Could you check a few things on this model? Use its own coordinates, in mm. Round coordinates to 2 decimals unless told otherwise and drop trailing zeros.
from build123d import *

# Parameters (mm, degrees)
F1_DEPTH = 4


# Not quite as in the source:
# - ends of sketch curves that miss each other by under 0.0002 mm in the source are joined


with BuildPart() as f1:
    # F0 (on Top) → F1 (new body)
    with BuildSketch(Plane.XY):
        with BuildLine():
            add(Edge.make_bspline(
                [(-23.29275, 188.71263), (-40.744167, 195.27633), (-59.410257, 198.41332), (-78.043821, 198.249744)],
                knots=[0, 0, 0, 0, 1, 1, 1, 1], degree=3))
            add(Edge.make_bspline(
                [(-78.043821, 198.249744), (-119.036105, 197.889891), (-160.001254, 181.57068), (-187.364696, 150.031637)],
                knots=[0, 0, 0, 0, 1, 1, 1, 1], degree=3))
            add(Edge.make_bspline(
                [(-187.364696, 150.031637), (-187.364865, 150.031442), (-187.364978, 150.031355), (-187.365261, 150.031072)],
                knots=[0, 0, 0, 0, 1, 1, 1, 1], degree=3))
            add(Edge.make_bspline(
                [(-187.365261, 150.031072), (-223.157197, 108.912672), (-239.83493, 53.349791), (-240.796196, -0.140351)],
                knots=[0, 0, 0, 0, 1, 1, 1, 1], degree=3))
            add(Edge.make_bspline(
                [(-240.796196, -0.140351), (-240.797267, -0.200062), (-240.797267, -0.259787), (-240.796196, -0.319498)],
                knots=[0, 0, 0, 0, 1, 1, 1, 1], degree=3))
            add(Edge.make_bspline(
                [(-240.796196, -0.319498), (-239.840937, -53.821863), (-222.970632, -108.900151), (-187.197127, -149.997041)],
                knots=[0, 0, 0, 0, 1, 1, 1, 1], degree=3))
            add(Edge.make_bspline(
                [(-187.197127, -149.997041), (-147.436926, -195.824596), (-79.112374, -209.648856), (-23.30153, -188.74031)],
                knots=[0, 0, 0, 0, 1, 1, 1, 1], degree=3))
            Line((-23.30153, -188.74031), (-23.130102, -188.679124))
            add(Edge.make_bspline(
                [(-23.130102, -188.679124), (1.059853, -180.570344), (21.278733, -165.037933), (38.938938, -147.973536)],
                knots=[0, 0, 0, 0, 1, 1, 1, 1], degree=3))
            add(Edge.make_bspline(
                [(38.938938, -147.973536), (52.026993, -136.892306), (62.204773, -123.641634), (75.896277, -117.517243)],
                knots=[0, 0, 0, 0, 1, 1, 1, 1], degree=3))
            add(Edge.make_bspline(
                [(75.896277, -117.517243), (83.85737, -115.06047), (91.397501, -116.61066), (99.542858, -119.902331)],
                knots=[0, 0, 0, 0, 1, 1, 1, 1], degree=3))
            add(Edge.make_bspline(
                [(99.542858, -119.902331), (107.756908, -123.2218), (116.195437, -128.328386), (125.148457, -131.870331)],
                knots=[0, 0, 0, 0, 1, 1, 1, 1], degree=3))
            add(Edge.make_bspline(
                [(125.148457, -131.870331), (132.727224, -134.996817), (140.627979, -137.381228), (148.394876, -139.826571)],
                knots=[0, 0, 0, 0, 1, 1, 1, 1], degree=3))
            add(Edge.make_bspline(
                [(148.394876, -139.826571), (148.394876, -139.826853), (148.397698, -139.826853), (148.397698, -139.826571)],
                knots=[0, 0, 0, 0, 1, 1, 1, 1], degree=3))
            add(Edge.make_bspline(
                [(148.397698, -139.826571), (148.40052, -139.826571), (148.401649, -139.829393), (148.403907, -139.829393)],
                knots=[0, 0, 0, 0, 1, 1, 1, 1], degree=3))
            add(Edge.make_bspline(
                [(148.403907, -139.829393), (172.528911, -147.473466), (202.043599, -149.701441), (222.443157, -131.039695)],
                knots=[0, 0, 0, 0, 1, 1, 1, 1], degree=3))
            Line((222.443157, -131.039695), (222.513713, -130.980174))
            add(Edge.make_bspline(
                [(222.513713, -130.980174), (229.464818, -125.631639), (234.197007, -117.510187), (235.635381, -108.839502)],
                knots=[0, 0, 0, 0, 1, 1, 1, 1], degree=3))
            add(Edge.make_bspline(
                [(235.635381, -108.839502), (237.078806, -100.138393), (234.900785, -90.513402), (227.492818, -83.846297)],
                knots=[0, 0, 0, 0, 1, 1, 1, 1], degree=3))
            add(Edge.make_bspline(
                [(227.492818, -83.846297), (227.400465, -83.76321), (227.305045, -83.683596), (227.206758, -83.607622)],
                knots=[0, 0, 0, 0, 1, 1, 1, 1], degree=3))
            add(Edge.make_bspline(
                [(227.206758, -83.607622), (220.687876, -78.567613), (213.176701, -75.418408), (207.090691, -71.705791)],
                knots=[0, 0, 0, 0, 1, 1, 1, 1], degree=3))
            add(Edge.make_bspline(
                [(207.090691, -71.705791), (201.005472, -67.993635), (196.586267, -64.15215), (194.627165, -57.863121)],
                knots=[0, 0, 0, 0, 1, 1, 1, 1], degree=3))
            add(Edge.make_bspline(
                [(194.627165, -57.863121), (194.626911, -57.862275), (194.627165, -57.86171), (194.627165, -57.860864)],
                knots=[0, 0, 0, 0, 1, 1, 1, 1], degree=3))
            add(Edge.make_bspline(
                [(194.627165, -57.860864), (190.811493, -45.539507), (200.792423, -32.097127), (214.099398, -32.108636)],
                knots=[0, 0, 0, 0, 1, 1, 1, 1], degree=3))
            add(Edge.make_bspline(
                [(214.099398, -32.108636), (214.100339, -32.108637), (214.10128, -32.108637), (214.10222, -32.108636)],
                knots=[0, 0, 0, 0, 1, 1, 1, 1], degree=3))
            add(Edge.make_bspline(
                [(214.10222, -32.108636), (222.998711, -32.113688), (230.233817, -27.742198), (234.609616, -21.595858)],
                knots=[0, 0, 0, 0, 1, 1, 1, 1], degree=3))
            add(Edge.make_bspline(
                [(234.609616, -21.595858), (238.985415, -15.449518), (240.879719, -7.737472), (240.796999, -0.090745)],
                knots=[0, 0, 0, 0, 1, 1, 1, 1], degree=3))
            add(Edge.make_bspline(
                [(240.796999, -0.090745), (240.714308, 7.555981), (238.653296, 15.239885), (234.273376, 21.375232)],
                knots=[0, 0, 0, 0, 1, 1, 1, 1], degree=3))
            add(Edge.make_bspline(
                [(234.273376, 21.375232), (229.893457, 27.51058), (222.80982, 31.975787), (214.131967, 32.074872)],
                knots=[0, 0, 0, 0, 1, 1, 1, 1], degree=3))
            add(Edge.make_bspline(
                [(214.131967, 32.074872), (200.3598011228, 32.409862366), (190.6341888263, 45.5397705426), (194.460767, 57.895973)],
                knots=[0.0012785739, 0.0012785739, 0.0012785739, 0.0012785739, 1, 1, 1, 1], degree=3))
            add(Edge.make_bspline(
                [(194.460767, 57.895973), (194.460993, 57.89682), (194.460767, 57.897384), (194.460767, 57.898231)],
                knots=[0, 0, 0, 0, 1, 1, 1, 1], degree=3))
            add(Edge.make_bspline(
                [(194.460767, 57.898231), (196.419841, 64.18724), (200.839074, 68.028874), (206.924293, 71.740898)],
                knots=[0, 0, 0, 0, 1, 1, 1, 1], degree=3))
            add(Edge.make_bspline(
                [(206.924293, 71.740898), (213.010274, 75.453396), (220.521421, 78.602146), (227.040331, 83.642189)],
                knots=[0, 0, 0, 0, 1, 1, 1, 1], degree=3))
            add(Edge.make_bspline(
                [(227.040331, 83.642189), (227.138629, 83.718163), (227.234058, 83.797777), (227.32642, 83.880865)],
                knots=[0, 0, 0, 0, 1, 1, 1, 1], degree=3))
            add(Edge.make_bspline(
                [(227.32642, 83.880865), (234.734386, 90.548), (236.91238, 100.173387), (235.468954, 108.87462)],
                knots=[0, 0, 0, 0, 1, 1, 1, 1], degree=3))
            add(Edge.make_bspline(
                [(235.468954, 108.87462), (234.0392708475, 117.493181786), (229.358044954, 125.5721274646), (222.4753975178, 130.9216294129)],
                knots=[0, 0, 0, 0, 0.9904989081, 0.9904989081, 0.9904989081, 0.9904989081], degree=3))
            add(Edge.make_bspline(
                [(222.4753975178, 130.9216294129), (202.2201967941, 149.6382929896), (173.4466709537, 148.1501016784), (149.669561, 140.174275)],
                knots=[0.0028310813, 0.0028310813, 0.0028310813, 0.0028310813, 1, 1, 1, 1], degree=3))
            add(Edge.make_bspline(
                [(149.669561, 140.174275), (147.849594, 139.64173), (141.739935, 137.657691), (138.376805, 136.671302)],
                knots=[0, 0, 0, 0, 1, 1, 1, 1], degree=3))
            add(Edge.make_bspline(
                [(138.376805, 136.671302), (138.337334, 136.659662), (138.298008, 136.647535), (138.258836, 136.634923)],
                knots=[0, 0, 0, 0, 1, 1, 1, 1], degree=3))
            add(Edge.make_bspline(
                [(138.258836, 136.634923), (130.579485, 134.174462), (132.826877, 134.841689), (125.095823, 131.950695)],
                knots=[0, 0, 0, 0, 1, 1, 1, 1], degree=3))
            add(Edge.make_bspline(
                [(125.095823, 131.950695), (125.066878, 131.939938), (125.038034, 131.928913), (125.009293, 131.917621)],
                knots=[0, 0, 0, 0, 1, 1, 1, 1], degree=3))
            add(Edge.make_bspline(
                [(125.009293, 131.917621), (116.046028, 128.375264), (107.599145, 123.260353), (99.376657, 119.937508)],
                knots=[0, 0, 0, 0, 1, 1, 1, 1], degree=3))
            add(Edge.make_bspline(
                [(99.376657, 119.937508), (91.231301, 116.645826), (83.69117, 115.095644), (75.730076, 117.5524)],
                knots=[0, 0, 0, 0, 1, 1, 1, 1], degree=3))
            add(Edge.make_bspline(
                [(75.730076, 117.5524), (62.038375, 123.676899), (51.860539, 136.927923), (38.772201, 148.009249)],
                knots=[0, 0, 0, 0, 1, 1, 1, 1], degree=3))
            add(Edge.make_bspline(
                [(38.772201, 148.009249), (21.11234, 165.071874), (0.895704, 180.602741), (-23.291056, 188.712066)],
                knots=[0, 0, 0, 0, 1, 1, 1, 1], degree=3))
            Line((-23.291056, 188.712066), (-23.29275, 188.71263))
        make_face()
        with BuildLine():
            add(Edge.make_bspline(
                [(222.4753975178, 130.9216294129), (222.4093775909, 130.9729430579), (222.3431551094, 131.0240055645), (222.276731, 131.074815)],
                knots=[0.9904989081, 0.9904989081, 0.9904989081, 0.9904989081, 1, 1, 1, 1], degree=3))
            add(Edge.make_bspline(
                [(222.647712, 130.761724), (222.5903427082, 130.8151888768), (222.5329044444, 130.8684905764), (222.4753975178, 130.9216294129)],
                knots=[0, 0, 0, 0, 0.0028310813, 0.0028310813, 0.0028310813, 0.0028310813], degree=3))
            Line((222.647712, 130.761724), (222.276731, 131.074815))
        make_face(mode=Mode.SUBTRACT)
        with BuildLine():
            add(Edge.make_bspline(
                [(222.647712, 130.761724), (222.5903427082, 130.8151888768), (222.5329044444, 130.8684905764), (222.4753975178, 130.9216294129)],
                knots=[0, 0, 0, 0, 0.0028310813, 0.0028310813, 0.0028310813, 0.0028310813], degree=3))
            add(Edge.make_bspline(
                [(222.4753975178, 130.9216294129), (222.4093775909, 130.9729430579), (222.3431551094, 131.0240055645), (222.276731, 131.074815)],
                knots=[0.9904989081, 0.9904989081, 0.9904989081, 0.9904989081, 1, 1, 1, 1], degree=3))
            Line((222.276731, 131.074815), (222.647712, 130.761724))
        make_face()
    extrude(amount=F1_DEPTH)


solid = f1.part
Item 1: If we section it at A-A, the plane x = 200: Count the separate pieces of the cut face and the enclosed holes in it, then the cut area to 3 significant figures.
Results list:
separate pieces: 3
enclosed holes: 0
area: 918 mm2
Item 2: Will these pins go through, and if not, where does the flat tip stop? pin 1 (2 mm diameter, centred on x = -182, y = 47.5, fed in from -Z); pin 2 (2 mm diameter, centred on x = 26, z = 3.5, fed in from +Y); pin 3 (1 mm diameter, centred on y = 61.5, z = 1.5, fed in from +X).
Results list:
pin 1: stops at z = 0
pin 2: stops at y = 160.45
pin 3: stops at x = 196.26
Item 3: If I drill on line 1 along Y through (x, z) = (-121.5, 3.5); line 2 along X through (y, z) = (-84, 3.5); line 3 along Y through (x, z) = (85, 0.6), over which ranges is the centre line in solid material (lowest first)?
Results list:
line 1: y = -191.71 to 191.74
line 2: x = -225.57 to 227.66
line 3: y = -116.33 to 116.38
